CAD build for the part. Positions are in the model's coordinates, mm. A direction names the side the tool comes from. Coordinates: 2 decimals unless noted, no trailing zeros. Write each loop counter-clockwise with the first axis right and the second up, starting at its lowest first coordinate (ties: lowest second). Pieces come first, ordered by that corner, then holes. Notation, with made-up numbers: (-18.5, 30.5) -> (28.5, 30.5) arc R26 cw to (28.5, 57.5) -> close; hole circle Ø3 at (-25.75, 2.5). An arc over 180 degrees is marked (long way). Answer as CSV lines item,"result".
```python
from build123d import *

# Parameters (mm, degrees)
F1_DEPTH = 10
F2_R     = 1
F3_R     = 2
F4_W     = 5
F4_H     = 5
F5_DEPTH = 10.25
F6_W     = 5
F6_H     = 5
F7_W     = 5
F7_H     = 5
F8_W     = 5
F8_H     = 5
F9_DEPTH = 5


with BuildPart() as f1:
    # F0 (on Top) → F1 (new body)
    with BuildSketch(Plane.XY):
        with BuildLine():
            ThreePointArc((4.8593298853, -14.4550826032), (4.4870695728, -13.259622802), (4.1751297651, -12.0470241738))
            ThreePointArc((4.1751297651, -12.0470241738), (0, -12.75), (-4.1751297651, -12.0470241738))
            ThreePointArc((-4.1751297651, -12.0470241738), (-4.4870695728, -13.259622802), (-4.8593298853, -14.4550826032))
            ThreePointArc((-4.8593298853, -14.4550826032), (-2.4619596159, -15.0499586328), (0, -15.25))
            ThreePointArc((0, -15.25), (2.4619596159, -15.0499586328), (4.8593298853, -14.4550826032))
        make_face()
        with BuildLine():
            ThreePointArc((0, -15.25), (-2.4619596159, -15.0499586328), (-4.8593298853, -14.4550826032))
            ThreePointArc((-4.8593298853, -14.4550826032), (-6.1206106512, -17.4986832949), (-7.7711643122, -20.35))
            Line((-7.7711643122, -20.35), (0, -20.35))
            Line((0, -20.35), (0, -15.25))
        make_face()
        with BuildLine():
            ThreePointArc((7.7711643122, -20.35), (6.1206106512, -17.4986832949), (4.8593298853, -14.4550826032))
            ThreePointArc((4.8593298853, -14.4550826032), (2.4619596159, -15.0499586328), (0, -15.25))
            Line((0, -15.25), (0, -20.35))
            Line((0, -20.35), (7.7711643122, -20.35))
        make_face()
        with BuildLine():
            ThreePointArc((-12.1977073115, -25.35), (-9.8167372296, -22.998464997), (-7.7711643122, -20.35))
            Line((-7.7711643122, -20.35), (-19.6810808999, -20.35))
            ThreePointArc((-19.6810808999, -20.35), (-24.6329372033, -22.4587536765), (-30, -22.8616926958))
            Line((-30, -22.8616926958), (-30, -25.35))
            Line((-30, -25.35), (-12.1977073115, -25.35))
        make_face()
        with BuildLine():
            Line((-30, -20.35), (-30, -22.8616926958))
            ThreePointArc((-30, -22.8616926958), (-24.6329372033, -22.4587536765), (-19.6810808999, -20.35))
            Line((-19.6810808999, -20.35), (-27.0704207387, -20.35))
            ThreePointArc((-27.0704207387, -20.35), (-28.5352103694, -20.4268397503), (-30, -20.35))
        make_face()
        with BuildLine():
            Line((0, -20.35), (-7.7711643122, -20.35))
            ThreePointArc((-7.7711643122, -20.35), (-9.8167372296, -22.998464997), (-12.1977073115, -25.35))
            Line((-12.1977073115, -25.35), (0, -25.35))
            Line((0, -25.35), (0, -20.35))
        make_face()
        with BuildLine():
            ThreePointArc((12.1977073115, -25.35), (9.8167372296, -22.998464997), (7.7711643122, -20.35))
            Line((7.7711643122, -20.35), (0, -20.35))
            Line((0, -20.35), (0, -25.35))
            Line((0, -25.35), (12.1977073115, -25.35))
        make_face()
        with BuildLine():
            Line((19.6810808999, -20.35), (7.7711643122, -20.35))
            ThreePointArc((7.7711643122, -20.35), (9.8167372296, -22.998464997), (12.1977073115, -25.35))
            Line((12.1977073115, -25.35), (30, -25.35))
            Line((30, -25.35), (30, -22.8616926958))
            ThreePointArc((30, -22.8616926958), (24.6329372033, -22.4587536765), (19.6810808999, -20.35))
        make_face()
        with BuildLine():
            Line((27.0704207387, -20.35), (19.6810808999, -20.35))
            ThreePointArc((19.6810808999, -20.35), (24.6329372033, -22.4587536765), (30, -22.8616926958))
            Line((30, -22.8616926958), (30, -20.35))
            ThreePointArc((30, -20.35), (28.5352103694, -20.4268397503), (27.0704207387, -20.35))
        make_face()
        with BuildLine():
            ThreePointArc((-12.0352103694, -6.4268397503), (-12.1363238462, -4.6029645348), (-12.438425012, -2.8014430604))
            ThreePointArc((-12.438425012, -2.8014430604), (-13.4233051179, 0.1973824432), (-14.9612028693, 2.9537956434))
            ThreePointArc((-14.9612028693, 2.9537956434), (-15.2486507313, -0.2028567877), (-14.8773319104, -3.3507454733))
            ThreePointArc((-14.8773319104, -3.3507454733), (-13.863287972, -6.3538765023), (-12.2503272762, -9.0825096547))
            ThreePointArc((-12.2503272762, -9.0825096547), (-12.0890775255, -7.7590238521), (-12.0352103694, -6.4268397503))
        make_face()
        with BuildLine():
            ThreePointArc((-4.8593298853, -14.4550826032), (-4.4870695728, -13.259622802), (-4.1751297651, -12.0470241738))
            ThreePointArc((-4.1751297651, -12.0470241738), (-9.5064579689, -8.4964555484), (-12.438425012, -2.8014430604))
            ThreePointArc((-12.438425012, -2.8014430604), (-12.1363238462, -4.6029645348), (-12.0352103694, -6.4268397503))
            ThreePointArc((-12.0352103694, -6.4268397503), (-12.0890775255, -7.7590238521), (-12.2503272762, -9.0825096547))
            ThreePointArc((-12.2503272762, -9.0825096547), (-8.9666731326, -12.3353667531), (-4.8593298853, -14.4550826032))
        make_face()
        with BuildLine():
            ThreePointArc((12.4384250802, -2.8014427577), (9.5064580723, -8.4964554327), (4.1751297651, -12.0470241738))
            ThreePointArc((4.1751297651, -12.0470241738), (4.4870695728, -13.259622802), (4.8593298853, -14.4550826032))
            ThreePointArc((4.8593298853, -14.4550826032), (8.9666731326, -12.3353667531), (12.2503272762, -9.0825096547))
            ThreePointArc((12.2503272762, -9.0825096547), (12.0426040821, -5.9329391), (12.4384250802, -2.8014427577))
        make_face()
        with BuildLine():
            ThreePointArc((14.9612028693, 2.9537956434), (13.4233051801, 0.1973825853), (12.4384250802, -2.8014427577))
            ThreePointArc((12.4384250802, -2.8014427577), (12.0426040821, -5.9329391), (12.2503272762, -9.0825096547))
            ThreePointArc((12.2503272762, -9.0825096547), (13.8632879655, -6.3538765165), (14.8773319036, -3.3507455038))
            ThreePointArc((14.8773319036, -3.3507455038), (15.1565466306, -1.6857028906), (15.25, 0))
            ThreePointArc((15.25, 0), (15.177628994, 1.4839400666), (14.9612028693, 2.9537956434))
        make_face()
        with BuildLine():
            ThreePointArc((-19.6810808999, -20.35), (-14.7609019356, -15.5108051385), (-12.2503272762, -9.0825096547))
            ThreePointArc((-12.2503272762, -9.0825096547), (-13.863287972, -6.3538765023), (-14.8773319104, -3.3507454733))
            ThreePointArc((-14.8773319104, -3.3507454733), (-14.621003629, -4.8793092054), (-14.5352103694, -6.4268397503))
            ThreePointArc((-14.5352103694, -6.4268397503), (-18.1307148307, -15.7941484666), (-27.0704207387, -20.35))
            Line((-27.0704207387, -20.35), (-19.6810808999, -20.35))
        make_face()
        with BuildLine():
            ThreePointArc((14.8773319036, -3.3507455038), (13.8632879655, -6.3538765165), (12.2503272762, -9.0825096547))
            ThreePointArc((12.2503272762, -9.0825096547), (14.7609019356, -15.5108051385), (19.6810808999, -20.35))
            Line((19.6810808999, -20.35), (27.0704207387, -20.35))
            ThreePointArc((27.0704207387, -20.35), (17.1590319273, -14.5866537221), (14.8773319036, -3.3507455038))
        make_face()
        with BuildLine():
            ThreePointArc((-12.438425012, -2.8014430604), (-12.6311834993, 1.7365780743), (-11.2209196713, 6.0542102482))
            Line((-11.2209196713, 6.0542102482), (-13.0527161264, 7.8860067033))
            ThreePointArc((-13.0527161264, 7.8860067033), (-14.2223975074, 5.5032634991), (-14.9612028693, 2.9537956434))
            ThreePointArc((-14.9612028693, 2.9537956434), (-13.4233051179, 0.1973824432), (-12.438425012, -2.8014430604))
        make_face()
        with BuildLine():
            Line((13.0527161264, 7.8860067033), (11.2209196713, 6.0542102482))
            ThreePointArc((11.2209196713, 6.0542102482), (12.3618207763, 3.1221606454), (12.75, 0))
            ThreePointArc((12.75, 0), (12.6718668667, -1.4093580502), (12.4384250802, -2.8014427577))
            ThreePointArc((12.4384250802, -2.8014427577), (13.4233051801, 0.1973825853), (14.9612028693, 2.9537956434))
            ThreePointArc((14.9612028693, 2.9537956434), (14.2223975074, 5.5032634991), (13.0527161264, 7.8860067033))
        make_face()
        with BuildLine():
            Line((-30, -25.85), (-12.7954249224, -25.85))
            ThreePointArc((-12.7954249224, -25.85), (-12.4946178162, -25.6023290673), (-12.1977073115, -25.35))
            Line((-12.1977073115, -25.35), (-30, -25.35))
            Line((-30, -25.35), (-30, -25.85))
        make_face()
        with BuildLine():
            ThreePointArc((12.7954249224, -25.85), (12.4946178162, -25.6023290673), (12.1977073115, -25.35))
            Line((12.1977073115, -25.35), (0, -25.35))
            Line((0, -25.35), (-12.1977073115, -25.35))
            ThreePointArc((-12.1977073115, -25.35), (-12.4946178162, -25.6023290673), (-12.7954249224, -25.85))
            Line((-12.7954249224, -25.85), (12.7954249224, -25.85))
        make_face()
        with BuildLine():
            Line((30, -25.35), (12.1977073115, -25.35))
            ThreePointArc((12.1977073115, -25.35), (12.4946178162, -25.6023290673), (12.7954249224, -25.85))
            Line((12.7954249224, -25.85), (30, -25.85))
            Line((30, -25.85), (30, -25.35))
        make_face()
    extrude(amount=F1_DEPTH)

    # F2
    f2_edges = [f1.edges().sort_by_distance(p)[0] for p in [
        (-7.771164, -20.35, 5),
        (-4.85933, -14.455083, 5),
        (-12.250327, -9.08251, 5),
        (-19.681081, -20.35, 5),
        (7.771164, -20.35, 5),
        (4.85933, -14.455083, 5),
        (12.250327, -9.08251, 5),
        (19.681081, -20.35, 5),
    ]]
    fillet(f2_edges, radius=F2_R)

    # F3
    f3_edges = [f1.edges().sort_by_distance(p)[0] for p in [
        (30, -20.35, 5),
        (-30, -20.35, 5),
    ]]
    fillet(f3_edges, radius=F3_R)

    # F4 (on face) → F5 (join)
    with BuildSketch(Plane.XZ.offset(25.85)):
        with Locations((-20, 2.5)):
            Rectangle(F4_W, F4_H)
        with Locations((0, 2.5)):
            Rectangle(F4_W, F4_H)
        with Locations((20, 2.5)):
            Rectangle(F4_W, F4_H)
    extrude(amount=F5_DEPTH)

    # F6 (on face) + F7 (on face) + F8 (on face) → F9 (join)
    with BuildSketch(Plane.XY.offset(5)):
        with Locations((-20, -33.6)):
            Rectangle(F6_W, F6_H)
    with BuildSketch(Plane.XY.offset(5)):
        with Locations((0, -33.6)):
            Rectangle(F7_W, F7_H)
    with BuildSketch(Plane.XY.offset(5)):
        with Locations((20, -33.6)):
            Rectangle(F8_W, F8_H)
    extrude(amount=F9_DEPTH)


solid = f1.part
```
Item 1: Flat gauge pins, fed straight in: pin 1 (1.5 mm diameter, centred on x = 20, z = 7.5, fed in from +Y); pin 2 (4 mm diameter, centred on x = 23.5, z = 8.5, fed in from +Y); pin 3 (2.5 mm diameter, centred on x = 19, y = -28, fed in from +Z); pin 4 (5 mm diameter, centred on x = 15.5, y = -24, fed in from -Z). Where does each tip first touch, or does it go through?
Answer below:
pin 1,"stops at y = -16.9"
pin 2,"stops at y = -18.53"
pin 3,"stops at z = 5"
pin 4,"stops at z = 0"
Item 2: Saw through at A-A on y = -33. Give the cut face in (x, z).
Answer below:
outline,"(-22.5, 0) -> (-17.5, 0) -> (-17.5, 10) -> (-22.5, 10) -> close; (-2.5, 0) -> (2.5, 0) -> (2.5, 10) -> (-2.5, 10) -> close; (17.5, 0) -> (22.5, 0) -> (22.5, 10) -> (17.5, 10) -> close"
Item 3: Two-plate mould, pull along Y, no slides. Class faces 5 (the flat face through (0, -36.1, 5)), 6 (the cylindrical face through (-8.6, -12.594, 4.93)), 7 (the flat face through (13, -20.35, 5)), 8 (the flat face through (-20, -34, 10)): pulls with the +Y half, pulls with the -Y half, needs draft (parallel to the pull), parting line crosses it, or undercut.
Answer below:
face 5,"pulls with the -Y half"
face 6,"undercut"
face 7,"undercut"
face 8,"needs draft"
Item 4: Wall check: line 1 (X direction, y = -32.5, z = 7); line 2 (Y direction, x = 0, z = 6); line 3 (X direction, y = 5, z = 7). Give the ranges that are in metal, low to high. Write a range as from..to.
Answer below:
line 1,"x = -22.5..-17.5, -2.5..2.5, 17.5..22.5"
line 2,"y = -36.1..-31.1, -25.85..-12.75"
line 3,"x = -14.41..-11.73, 11.73..14.41"
Item 5: Saw through at B-B on y = -4. Give the cut face in (x, z).
Answer below:
outline,"(-14.75, 0) -> (-12.11, 0) -> (-12.11, 10) -> (-14.75, 10) -> close; (12.11, 0) -> (14.75, 0) -> (14.75, 10) -> (12.11, 10) -> close"
Item 6: 3-axis set-ups, long thin cutter, end or side, ignore diameter. For faces 1 (the flat face through (-17.5, -32, 4)), 2 (the cylindrical face through (6.24, -17.74, 4.93)), 3 (the flat face through (-22.5, -32, 4)), 4 (the flat face through (0, -31.1, 7)): which of +Z, -Z, +X, -X, +Y, -Y reach the whole face in a straight line?
Answer below:
face 1,"+Z, -Z, -Y"
face 2,"+Z, -Z"
face 3,"+Z, -Z, -X, -Y"
face 4,"+Z, +X, -X"
Item 7: Saw through at C-C on z = 8. State how many separate pieces and enclosed holes the cut face has, and give its area (3 significant figures).
Answer below:
separate pieces,"4"
enclosed holes,"2"
area,"707 mm2"
